from build123d import *

# Parameters (mm, degrees)
F0_W     = 100
F0_H     = 100
F0_R     = 4
F1_DEPTH = 18
F3_DEPTH = 12
F4_R     = 10
F5_DEPTH = 30


with BuildPart() as f1:
    # F0 (on Front) → F1 (new body)
    with BuildSketch(Plane.XZ):
        Rectangle(F0_W, F0_H)
        with Locations((-40, -40)):
            Circle(F0_R, mode=Mode.SUBTRACT)
        with Locations((40, -40)):
            Circle(F0_R, mode=Mode.SUBTRACT)
        with Locations((-40, 40)):
            Circle(F0_R, mode=Mode.SUBTRACT)
        with Locations((40, 40)):
            Circle(F0_R, mode=Mode.SUBTRACT)
    extrude(amount=F1_DEPTH)

    # F2 (on face) → F3 (join)
    with BuildSketch(Plane.XZ.offset(18)):
        with BuildLine():
            Line((20, 35), (-20, 35))
            ThreePointArc((-20, 35), (-30.606602, 30.606602), (-35, 20))
            Line((-35, 20), (-35, -20))
            ThreePointArc((-35, -20), (-30.606602, -30.606602), (-20, -35))
            Line((-20, -35), (20, -35))
            ThreePointArc((20, -35), (30.606602, -30.606602), (35, -20))
            Line((35, -20), (35, 20))
            ThreePointArc((35, 20), (30.606602, 30.606602), (20, 35))
        make_face()
        with BuildLine():
            ThreePointArc((-30, 20), (-27.071068, 27.071068), (-20, 30))
            Line((-20, 30), (20, 30))
            ThreePointArc((20, 30), (27.071068, 27.071068), (30, 20))
            Line((30, 20), (30, -20))
            ThreePointArc((30, -20), (27.071068, -27.071068), (20, -30))
            Line((20, -30), (-20, -30))
            ThreePointArc((-20, -30), (-27.071068, -27.071068), (-30, -20))
            Line((-30, -20), (-30, 20))
        make_face(mode=Mode.SUBTRACT)
    extrude(amount=F3_DEPTH)

    # F4 (on face) → F5 (cut)
    with BuildSketch(Plane.XZ.offset(18)):
        Circle(F4_R)
    extrude(amount=-F5_DEPTH, mode=Mode.SUBTRACT)


solid = f1.part
Build history of the part. All positions in model axes, mm. A direction names the side the tool comes from. Give positions to 0.01 mm unless a question says otherwise; leave off trailing zeros. Order: outer loops, then holes, each group sorted by start corner. A loop starts at its lowest first (then second) coordinate and runs counter-clockwise, first axis right, second up. Notation, with made-up numbers: M 44.25,9.5 L 79.25,9.5 A6 ccw 79.25,13.5 Z; hole C -21,57.5 d7. An arc over 180 degrees is marked long. Use one line per item in the form item = value.
1) Drop flat-ended pins along their axis: pin 1 (6.5 mm diameter, centred on x = -40, z = 40, fed in from -Y); pin 2 (2 mm diameter, centred on x = -15.5, z = 29.5, fed in from -Y); pin 3 (12 mm diameter, centred on y = -25.5, z = -32, fed in from -X); pin 4 (9 mm diameter, centred on x = 40, z = 40, fed in from -Y). Give the stop position or say it passes through.
Calculated:
pin_1 = through
pin_2 = -30
pin_3 = -33.75
pin_4 = -18
2) Saw through at D-D (z = 0). Give the cut face in (x, y), plus the area to 3 significant figures.
Calculated:
outline = M -50,-18 L -35,-18 L -35,-30 L -30,-30 L -30,-18 L -10,-18 L -10,0 L -50,0 Z; M 10,-18 L 30,-18 L 30,-30 L 35,-30 L 35,-18 L 50,-18 L 50,0 L 10,0 Z
area = 1,560 mm2
3) Saw through at C-C (y = -19.25). Give the cut face in (x, z), plus the area to 3 significant figures.
Calculated:
outline = M -35,-20 A15 ccw -20,-35 L 20,-35 A15 ccw 35,-20 L 35,20 A15 ccw 20,35 L -20,35 A15 ccw -35,20 Z; hole M -30,-20 A10 ccw -20,-30 L 20,-30 A10 ccw 30,-20 L 30,20 A10 ccw 20,30 L -20,30 A10 ccw -30,20 Z
area = 1,190 mm2
4) Saw through at B-B (x = 0). Give the cut face in (y, z), plus the area to 3 significant figures.
Calculated:
outline = M -30,-35 L -18,-35 L -18,-50 L 0,-50 L 0,-10 L -18,-10 L -18,-30 L -30,-30 Z; M -30,30 L -18,30 L -18,10 L 0,10 L 0,50 L -18,50 L -18,35 L -30,35 Z
area = 1,560 mm2
5) Saw through at A-A (z = -40). Give the cut face in (x, y).
Calculated:
outline = M -50,-18 L -44,-18 L -44,0 L -50,0 Z; M -36,-18 L 36,-18 L 36,0 L -36,0 Z; M 44,-18 L 50,-18 L 50,0 L 44,0 Z
6) Two-plate mould, pull along Z, no slides. Class faces 1 (the face through (-35, -24, 0)), 2 (the face through (39.479, -8.874, -36.034)), 3 (the face through (-30.49, -23.92, 30.72)), 4 (the face through (-1, -9, -50)): released by +Z, released by -Z, zero draft, split by the parting line, or undercut.
Calculated:
face_1 = zero draft
face_2 = undercut
face_3 = released by +Z
face_4 = released by -Z
7) Probe probe 1 along Z at (x, y) = (40, -5); probe 2 along X at (y, z) = (-13.25, 41.5); probe 3 along X at (y, z) = (-15, 36.5). List the from-to ranges inside material, lowest first.
Calculated:
probe_1 = -50 to -44, -36 to 36, 44 to 50
probe_2 = -50 to -43.71, -36.29 to 36.29, 43.71 to 50
probe_3 = -50 to -41.94, -38.06 to 38.06, 41.94 to 50
8) Tool access for faces 5 (the face through (30.49, -23.92, -30.72)), 6 (the face through (-45, -18, 1)), 7 (the face through (0, -24, 35)): list every direction of +Z, -Z, +X, -X, +Y, -Y with a clear straight run to the whole face (end or side of a thin tool).
Calculated:
face_5 = -Z, +X, -Y
face_6 = -Y
face_7 = +Z, +X, -X, -Y
